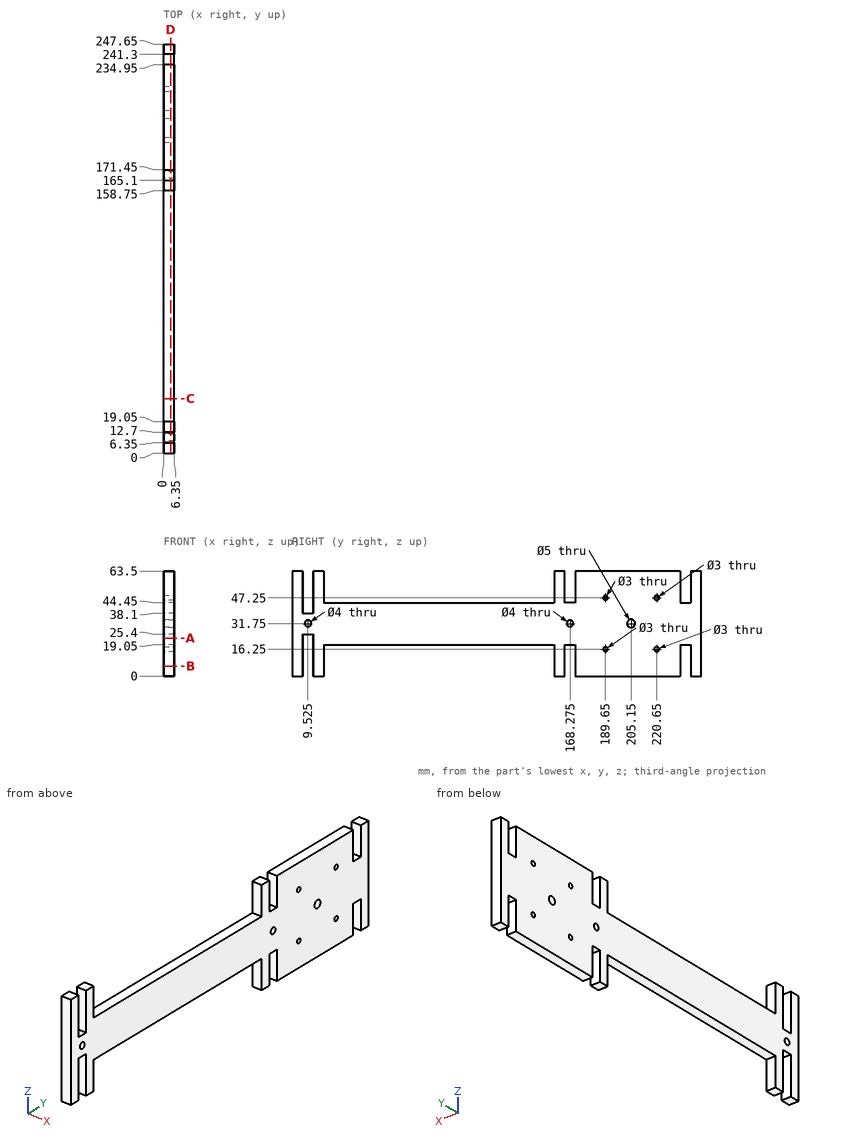
The drawing under review shows one solid part. Ordinate dimensions are in mm from its lowest x, y, z. Round coordinates to 2 decimals unless told otherwise and drop trailing zeros. Order: outer loops, then holes, each group sorted by start corner. A loop starts at its lowest first (then second) coordinate and runs counter-clockwise, first axis right, second up. Notation, with made-up numbers: M -8,72.5 L 13,72.5 A6 ccw 13,80.5 Z; hole C 52,-34 d6. An arc over 180 degrees is marked long. Answer as CSV lines item,"result". Start each with the question number.
1) Wall thickness on line 1 along Y through (x, z) = (3, 31.75) (3 decimals); line 2 along Y through (x, z) = (4, 18); line 3 along Y through (x, z) = (5.5, 22.5): over which ranges is each line inside the solid? List them lowest first. Write a range as [from, to].
2) Add section A-A (z = 23). Give the boundary of the cut face in (x, y), then the cut area to 3 significant figures.
3) Add section D-D (x = 4.25). Give the number of separate pieces and of enclosed holes in the cut face, then the cut area to 3 significant figures.
4) For pin 1 Ø6.5 at (y, z) = (168.275, 31.75) entering from -X; pin 2 Ø1.9 at (x, y) = (4, 239) entering from +Z; pin 3 Ø10 at (y, z) = (25, 7) entering from -X, all flat-tipped, find the tip position at first contact; note any pin that passes through.
5) Add section C-C (y = 33). Give the boundary of the cut face in (x, z), then the cut area to 3 significant figures.
6) Add section B-B (z = 6). Give the boundary of the cut face in (x, y), then the cut area to 3 significant figures.
Resolved:
1,line 1,"[0, 7.525], [11.525, 166.275], [170.275, 202.65], [207.65, 247.65]"
1,line 2,"[0, 6.35], [12.7, 19.05], [158.75, 165.1], [171.45, 234.95], [241.3, 247.65]"
1,line 3,"[0, 6.35], [12.7, 247.65]"
2,outline,"M 0,0 L 6.35,0 L 6.35,6.35 L 0,6.35 Z; M 0,12.7 L 6.35,12.7 L 6.35,247.65 L 0,247.65 Z"
2,area,"1,530 mm^2"
3,separate pieces,"1"
3,enclosed holes,"7"
3,area,"9,520 mm^2"
4,pin 1,"x = 0"
4,pin 2,"z = 44.45"
4,pin 3,"through"
5,outline,"M 0,19.05 L 6.35,19.05 L 6.35,44.45 L 0,44.45 Z"
5,area,"161 mm^2"
6,outline,"M 0,0 L 6.35,0 L 6.35,6.35 L 0,6.35 Z; M 0,12.7 L 6.35,12.7 L 6.35,19.05 L 0,19.05 Z; M 0,158.75 L 6.35,158.75 L 6.35,165.1 L 0,165.1 Z; M 0,171.45 L 6.35,171.45 L 6.35,234.95 L 0,234.95 Z; M 0,241.3 L 6.35,241.3 L 6.35,247.65 L 0,247.65 Z"
6,area,"565 mm^2"
